Work out the finished part from the listing and answer in its coordinate system (mm). A direction names the side the tool comes from. Give positions to 0.01 mm unless a question says otherwise; leave off trailing zeros. Order: outer loops, then holes, each group sorted by start corner. A loop starts at its lowest first (then second) coordinate and runs counter-clockwise, first axis right, second up. Notation, with made-up numbers: (-34, 78.5) - (-8, 78.5) arc R13 cw to (-8, 102.5) - close; hole circle Ø7 at (28, 55.25). An arc over 180 degrees is marked (long way). Put each result on its own line as item: value.
```python
from build123d import *

# Parameters (mm, degrees)
SKETCH1_R           = 8
BOSS_EXTRUDE1_DEPTH = 3
SKETCH2_R           = 3.9
BOSS_EXTRUDE2_DEPTH = 7
SKETCH3_R           = 1.15
CUT_EXTRUDE3_DEPTH  = 12
CUT_EXTRUDE4_DEPTH  = 3
FILLET1_R           = 0.7
FILLET2_R           = 0.5
FILLET3_R           = 0.5


with BuildPart() as part:
    # Sketch1 → Boss-Extrude1 (new body)
    with BuildSketch(Plane(origin=(0, 0, 0), x_dir=(1, 0, 0), z_dir=(0, 1, 0))):
        Circle(SKETCH1_R)
    extrude(amount=BOSS_EXTRUDE1_DEPTH)

    # Sketch2 → Boss-Extrude2 (add)
    with BuildSketch(Plane.XZ):
        Circle(SKETCH2_R)
    extrude(amount=BOSS_EXTRUDE2_DEPTH)

    # Sketch3 → Cut-Extrude3 (cut)
    with BuildSketch(Plane.XZ.offset(7)):
        Circle(SKETCH3_R)
    extrude(amount=-CUT_EXTRUDE3_DEPTH, mode=Mode.SUBTRACT)

    # Sketch6 → Cut-Extrude4 (cut)
    with BuildSketch(Plane(origin=(0, 3, 0), x_dir=(1, 0, 0), z_dir=(0, 1, 0))):
        Polygon((0, 2.540341184), (-2.2, 1.270170592), (-2.2, -1.270170592), (0, -2.540341184), (2.2, -1.270170592), (2.2, 1.270170592), align=None)
    extrude(amount=-CUT_EXTRUDE4_DEPTH, mode=Mode.SUBTRACT)

    # Fillet1
    fillet1_edges = [part.edges().sort_by_distance(p)[0] for p in [
        (1.1, 3, -1.905255888),
        (-1.1, 3, -1.905255888),
        (-2.2, 3, 0),
        (-1.1, 3, 1.905255888),
        (1.1, 3, 1.905255888),
        (2.2, 3, 0),
    ]]
    fillet(fillet1_edges, radius=FILLET1_R)

    # Fillet2
    fillet2_edges = [part.edges().sort_by_distance(p)[0] for p in [
        (-1.15, -7, 0),
    ]]
    fillet(fillet2_edges, radius=FILLET2_R)

    # Fillet3
    fillet3_edges = [part.edges().sort_by_distance(p)[0] for p in [
        (-8, 0, 0),
        (-3.9, 0, 0),
    ]]
    fillet(fillet3_edges, radius=FILLET3_R)


solid = part.part
```
(1) Determine the mould class of faces 4 (the face through (-1.226, 2.8, -2.076)), 5 (the face through (3.4, 3, -0.1)), 6 (the face through (-2.87, -3.7, 2.64)), 7 (the face through (-1.115, 1.166, 1.896)) for opening direction Z: pulls with the +Z half, pulls with the -Z half, needs draft (parallel to the pull), parting line crosses it, or undercut.
Geometry check:
face 4: undercut
face 5: needs draft
face 6: parting line crosses it
face 7: undercut
(2) Section A-A, the plane z = 0 is taken. Write down the section's boundary in (x, y).
Geometry check:
outline: (-8, 0.5) arc R0.5 ccw to (-7.5, 0) - (-4.4, 0) arc R0.5 cw to (-3.9, -0.5) - (-3.9, -7) - (-1.65, -7) arc R0.5 ccw to (-1.15, -6.5) - (-1.15, 0) - (-2.2, 0) - (-2.2, 2.3) arc R0.7 ccw to (-2.9, 3) - (-8, 3) - close; (1.15, -6.5) arc R0.5 ccw to (1.65, -7) - (3.9, -7) - (3.9, -0.5) arc R0.5 cw to (4.4, 0) - (7.5, 0) arc R0.5 ccw to (8, 0.5) - (8, 3) - (2.9, 3) arc R0.7 ccw to (2.2, 2.3) - (2.2, 0) - (1.15, 0) - close
(3) Section B-B, the plane y = -1.5 is taken. Write down the section's boundary in (x, z).
Geometry check:
outline: circle Ø7.8 at (0, 0); hole circle Ø2.3 at (0, 0)
(4) A tool of negligible diameter and unlimited length cuts with its end or side. For faces 1 (the face through (3.23, 0, 3.23)), 2 (the face through (1.115, 1.166, -1.896)), 3 (the face through (-1.73, 1.73, 7.81)), from which of +Z, -Z, +X, -X, +Y, -Y can it reach the whole face along a straight path? Write none if from no direction.
Geometry check:
face 1: -Y
face 2: +Y
face 3: +Y, -Y
(5) Given pin 1 (3 mm diameter, centred on x = -1.5, y = -2, fed in from -Z); pin 2 (2 mm diameter, centred on x = 0, z = -1, fed in from +Y); pin 3 (1.5 mm diameter, centred on x = 3.5, y = 1, fed in from +Z), each flat-ended and moving along its own axis, determine where each tip first touches the part or whether it passes through.
Geometry check:
pin 1: stops at z = -3.9
pin 2: stops at y = 0
pin 3: stops at z = 7.51
(6) Straight lines are drawn through the part: line 1 (Z direction, x = 0, y = -4.25); line 2 (Y direction, x = -3.5, z = -5.75); line 3 (Z direction, x = -2, y = 2.25). For each, find the intervals that lie inside material, in ascending order.
Geometry check:
line 1: z = -3.9 to -1.15, 1.15 to 3.9
line 2: y = 0 to 3
line 3: z = -7.75 to -1.39, 1.39 to 7.75
